Geometry check sheet. Reference: drawing and pictorial views, mm from the part's lowest x, y, z. A direction names the side the tool comes from. Give positions to 0.01 mm unless a question says otherwise; leave off trailing zeros. Loops run counter-clockwise (first coordinate to the right, second up) from the corner with the lowest first, then second, coordinate; pieces in that order, holes last. Notation, with made-up numbers: (68, -39) -> (111, -39) arc R30 cw to (111, -11) -> close; hole circle Ø2 at (71.25, 69). An arc over 180 degrees is marked (long way). Write item = value, one per line. Start each with the question number.
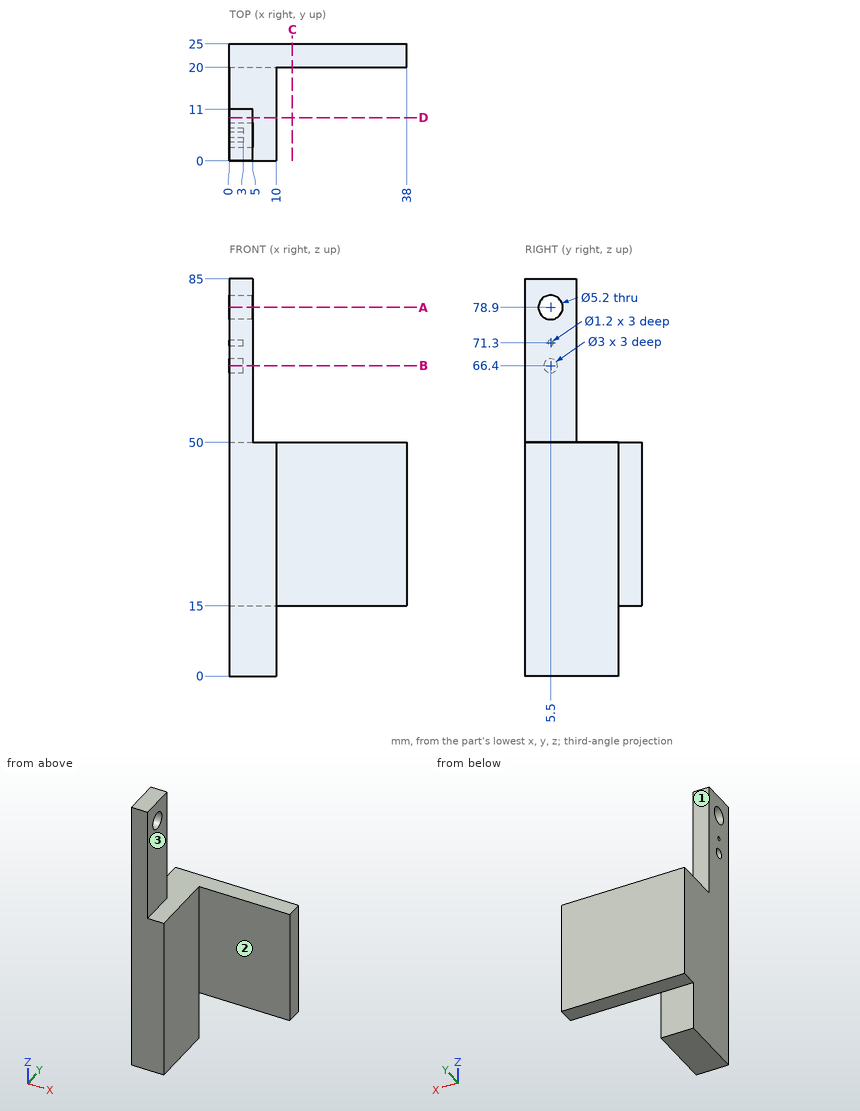
1) Depth check by flat-ended pin: pin 1 Ø8 at (y, z) = (3, 11.5) entering from -X; pin 2 Ø22.5 at (x, z) = (21.5, 39.5) entering from -Y; pin 3 Ø3.5 at (y, z) = (3.5, 62) entering from +X; pin 4 Ø5.5 at (x, z) = (2.5, 62) entering from +Y. Enter the tip coordinate at first touch or a pass-through.
2) Section check C-C (x = 13.5). Enter the section's corners in (y, z), plus the area to 3 significant figures.
3) Section check D-D (y = 9.25). Enter the section's corners in (x, z), plus the area to 3 significant figures.
4) Thickness scan on line 1 (Y direction, x = 0.7, z = 71.3); line 2 (X direction, y = 6.5, z = 65.5); line 3 (X direction, y = 4.25, z = 33.5). Record the ranges inside material, lowest first.
5) Tool access check on the marked faces 1, 2 and 3. Record the directions out of +Z, -Z, +X, -X, +Y, -Y that give a thin tool (end or side, any length) a straight path to the whole face; none if there is none.
6) Section check A-A (z = 78.9). Enter the section's corners in (x, y).
7) Section check B-B (z = 66.4). Enter the section's corners in (x, y).
Check result:
q1.pin_1 = 0
q1.pin_2 = 20
q1.pin_3 = 5
q1.pin_4 = 11
q2.outline = (20, 15) -> (25, 15) -> (25, 50) -> (20, 50) -> close
q2.area = 175 mm2
q3.outline = (0, 0) -> (10, 0) -> (10, 50) -> (5, 50) -> (5, 85) -> (0, 85) -> close
q3.area = 675 mm2
q4.line_1 = 0 to 4.9, 6.1 to 11
q4.line_2 = 3 to 5
q4.line_3 = 0 to 10
q5.face_1 = +Z, +X, -X, +Y
q5.face_2 = +Z, -Z, +X, -Y
q5.face_3 = +Z, +X, +Y, -Y
q6.outline = (0, 0) -> (5, 0) -> (5, 2.9) -> (0, 2.9) -> close; (0, 8.1) -> (5, 8.1) -> (5, 11) -> (0, 11) -> close
q7.outline = (0, 0) -> (5, 0) -> (5, 11) -> (0, 11) -> (0, 7) -> (3, 7) -> (3, 4) -> (0, 4) -> close
